Geometry: final body of the model. Coordinates: model frame, mm. A direction names the side the tool comes from. Coordinates: 2 decimals unless noted, no trailing zeros. Order: outer loops, then holes, each group sorted by start corner. A loop starts at its lowest first (then second) coordinate and runs counter-clockwise, first axis right, second up. Notation, with made-up numbers: (47.5, 12) -> (104.5, 12) arc R35 cw to (104.5, 46) -> close; hole circle Ø10 at (69, 34.5). An arc over 180 degrees is marked (long way). Use CSV: the item, a comma, the result in double quotes. Start each with the question number.
from build123d import *

# Parameters (mm, degrees)
SKETCH1_R               = 13
BOSS_EXTRUDE1_DEPTH     = 2
SKETCH2_R               = 11.5
BOSS_EXTRUDE2_DEPTH     = 1.5
SKETCH3_R               = 13
BOSS_EXTRUDE4_DEPTH     = 10
CUT_EXTRUDE1_DEPTH      = 7
CUT_EXTRUDE1_DEPTH_BACK = 23.808989456
CHAMFER1_SIZE           = 2
FILLET1_R               = 3


with BuildPart() as part:
    # Sketch1 → Boss-Extrude1 (new body)
    with BuildSketch(Plane(origin=(0, 0, 0), x_dir=(1, 0, 0), z_dir=(0, 1, 0))):
        with Locations(Location((0, 0, 0), (0, 0, 270))):
            Circle(SKETCH1_R)
    extrude(amount=BOSS_EXTRUDE1_DEPTH)

    # Sketch2 → Boss-Extrude2 (add)
    with BuildSketch(Plane(origin=(0, 2, 0), x_dir=(1, 0, 0), z_dir=(0, 1, 0))):
        with Locations(Location((0, 0, 0), (0, 0, 270))):
            Circle(SKETCH2_R)
    extrude(amount=BOSS_EXTRUDE2_DEPTH)

    # Sketch3 → Boss-Extrude4 (add)
    with BuildSketch(Plane(origin=(0, 3.5, 0), x_dir=(1, 0, 0), z_dir=(0, 1, 0))):
        with Locations(Location((0, 0, 0), (0, 0, 270))):
            Circle(SKETCH3_R)
    extrude(amount=BOSS_EXTRUDE4_DEPTH)

    # Sketch4 → Cut-Extrude1 (cut, two sides: drawn at the far end of the back side and taken through both)
    with BuildSketch(Plane(origin=(0, 0, 0), x_dir=(0, 0, -1), z_dir=(1, 0, 0)).offset(-CUT_EXTRUDE1_DEPTH_BACK)):
        Polygon((-0.040911755, 5.5), (-8.040911755, 5.5), (-4, 13.5), (0, 13.5), (4, 13.5), (7.959088245, 5.5), align=None)
    extrude(amount=CUT_EXTRUDE1_DEPTH + CUT_EXTRUDE1_DEPTH_BACK, mode=Mode.SUBTRACT)

    # Chamfer1
    # the kernel refuses this chamfer: 2 mm, written as the material it takes off along each edge
    with BuildSketch(Plane(origin=(0, 3.5, 0), x_dir=(0, 0, 1), z_dir=(-1, 0, 0))) as chamfer1_piece_1_section:
        Polygon((13, CHAMFER1_SIZE), (13 - CHAMFER1_SIZE, 0), (13, 0), align=None)
    chamfer1_piece_1 = revolve(axis=Axis((0, 3.5, 0), (0, 1, 0)), mode=Mode.PRIVATE)
    chamfer1_piece_1 = chamfer1_piece_1 - Plane(origin=(0, 4.739987211, 0), x_dir=(0, 0, 1), z_dir=(0, -1, 0)) * Cylinder(11.5, 52, mode=Mode.PRIVATE)
    add(chamfer1_piece_1, mode=Mode.SUBTRACT)

    # Fillet1
    fillet1_edges = [part.edges().sort_by_distance(p)[0] for p in [
        (13, 13.5, 0),
    ]]
    fillet(fillet1_edges, radius=FILLET1_R)


solid = part.part
(1) Line query: line 1 (Y direction, x = 5.25, z = -3); line 2 (Z direction, x = 1.75, y = 10.5); line 3 (Y direction, x = -10.75, z = 7). Output: solid intervals per line, ascending. Write a range as from..to.
(2) Section C-C (y = 7.75). Return loops of the section in (x, z).
(3) Section D-D (y = 11). Return loops of the section in (x, z).
(4) Access query for faces 1 (the face through (7, 9, 0)), 2 (the face through (13, 8, 0)), 3 (the face through (-11, 2, 5)). Directions: +Z, -Z, +X, -X, +Y, -Y. A direction counts if a zero-diameter tool reaches every point of the face in a straight line with its end or side. Return the directions, or none.
(5) First-contact query: pin 1 (1.5 mm diameter, centred on y = 7.5, z = -8.5, fed in from +X); pin 2 (1.5 mm diameter, centred on y = 10, z = 1, fed in from +X); pin 3 (3 mm diameter, centred on x = -9, y = 2.5, fed in from +Z). Flat tips, straight axial feed; report the tip coordinate or a pass-through.
(6) Section A-A (z = 0). Return loops of the section in (x, y).
(7) Mould query, pull axis Y, two halves, no side actions, for faces 4 (the face through (0.6, 13.5, 4.3)), 5 (the face through (-7.91, 0.986, -10.316)), 6 (the face through (-3, 5.5, 0)), 7 (the face through (-2.56, 9.44, 6.05)). Classes: pulls with the +Y half, pulls with the -Y half, needs draft (parallel to the pull), parting line crosses it, or undercut.
(8) Section B-B (x = 0). Return loops of the section in (y, z).
Check sheet entries:
1,line 1,"y = 0..5.5"
1,line 2,"z = -12.88..-5.48, 5.52..12.88"
1,line 3,"y = 0..2, 5.33..5.5, 7.56..11.5"
2,outline,"(-11.05, -6.85) arc R13 ccw (long way) to (-11.01, 6.9) -> (7, 6.9) -> (7, -6.85) -> close"
3,outline,"(-11.85, -5.24) arc R12.96 ccw (long way) to (-11.84, 5.26) -> (7, 5.26) -> (7, -5.24) -> close"
4,face 1,"-X"
4,face 2,"+Y, -Y"
4,face 3,"none"
5,pin 1,"stops at x = 10.44"
5,pin 2,"stops at x = 13"
5,pin 3,"stops at z = 10.56"
6,outline,"(-13, 0) -> (13, 0) -> (13, 2) -> (11.5, 2) -> (11.5, 4) -> (13, 5.5) -> (13, 10.5) arc R3 ccw to (10, 13.5) -> (7, 13.5) -> (7, 5.5) -> (-13, 5.5) -> (-11.5, 4) -> (-11.5, 2) -> (-13, 2) -> close"
7,face 4,"pulls with the +Y half"
7,face 5,"needs draft"
7,face 6,"undercut"
7,face 7,"undercut"
8,outline,"(0, -13) -> (2, -13) -> (2, -11.5) -> (4, -11.5) -> (5.5, -13) -> (10.5, -13) arc R3 ccw to (13.5, -10) -> (13.5, -4) -> (5.5, -7.96) -> (5.5, 8.04) -> (13.5, 4) -> (13.5, 10) arc R3 ccw to (10.5, 13) -> (5.5, 13) -> (4, 11.5) -> (2, 11.5) -> (2, 13) -> (0, 13) -> close"
